```python
from build123d import *

# Parameters (mm, degrees)
SKETCH_1_W          = 100
SKETCH_1_H          = 60
EXTRUDE_1_DEPTH     = 20
SKETCH_2_W          = 90
SKETCH_2_H          = 50
CUT_EXTRUDE_1_DEPTH = 15
CUT_EXTRUDE_6_DEPTH = 200
SKETCH_9_R          = 5
CUT_EXTRUDE_7_DEPTH = 2
CUT_EXTRUDE_START   = -2
SKETCH_10_R         = 5
CUT_EXTRUDE_8_DEPTH = 2
SKETCH_11_W         = 30
SKETCH_11_H         = 3.05
EXTRUDE_2_DEPTH     = 4
SKETCH_12_W         = 30
SKETCH_12_H         = 3.05
EXTRUDE_3_DEPTH     = 4


with BuildPart() as part:
    # 草图1 → 凸台-拉伸1 (new body)
    with BuildSketch(Plane(origin=(0, 0, 0), x_dir=(1, 0, 0), z_dir=(0, 1, 0))):
        with Locations((29.550198358, -13.555421679)):
            Rectangle(SKETCH_1_W, SKETCH_1_H)
    extrude(amount=EXTRUDE_1_DEPTH)

    # 草图2 → 切除-拉伸1 (cut)
    with BuildSketch(Plane.XZ):
        with Locations((29.550198358, 13.555421679)):
            Rectangle(SKETCH_2_W, SKETCH_2_H)
    extrude(amount=-CUT_EXTRUDE_1_DEPTH, mode=Mode.SUBTRACT)

    # 草图8 → 切除-拉伸6 (cut)
    with BuildSketch(Plane.XY.offset(43.555421679)):
        with BuildLine():
            ThreePointArc((32.150198358, 10), (31.388675989, 11.838477631), (29.550198358, 12.6))
            Line((29.550198358, 12.6), (29.550198358, 7.4))
            ThreePointArc((29.550198358, 7.4), (31.388675989, 8.161522369), (32.150198358, 10))
        make_face()
        with BuildLine():
            Line((29.550198358, 7.4), (29.550198358, 12.6))
            ThreePointArc((29.550198358, 12.6), (26.950198358, 10), (29.550198358, 7.4))
        make_face()
    extrude(amount=-CUT_EXTRUDE_6_DEPTH, mode=Mode.SUBTRACT)

    # 草图9 → 切除-拉伸7 (cut)
    with BuildSketch(Plane.XY.offset(-11.444578321)):
        with Locations((29.550198358, 10)):
            Circle(SKETCH_9_R)
    extrude(amount=-CUT_EXTRUDE_7_DEPTH, mode=Mode.SUBTRACT)

    # 草图10 → 切除-拉伸8 (cut)
    with BuildSketch(Plane(origin=(0, 0, 38.555421679), x_dir=(-1, 0, 0), z_dir=(0, 0, -1)).offset(CUT_EXTRUDE_START)):
        with Locations(Location((-29.550198358, 10, 0), (0, 0, 180))):
            Circle(SKETCH_10_R)
    extrude(amount=CUT_EXTRUDE_8_DEPTH, mode=Mode.SUBTRACT)

    # 草图11 → 凸台-拉伸2 (add)
    with BuildSketch(Plane(origin=(0, 0, -16.444578321), x_dir=(-1, 0, 0), z_dir=(0, 0, -1))):
        with Locations((5.449801642, 8.475)):
            Rectangle(SKETCH_11_W, SKETCH_11_H)
        with Locations((5.449801642, 11.525)):
            Rectangle(SKETCH_11_W, SKETCH_11_H)
        with Locations((-64.550198358, 8.475)):
            Rectangle(SKETCH_11_W, SKETCH_11_H)
        with Locations((-64.550198358, 11.525)):
            Rectangle(SKETCH_11_W, SKETCH_11_H)
    extrude(amount=EXTRUDE_2_DEPTH)

    # 草图12 → 凸台-拉伸3 (add)
    with BuildSketch(Plane.XY.offset(43.555421679)):
        with Locations((-5.449801642, 11.525)):
            Rectangle(SKETCH_12_W, SKETCH_12_H)
        with Locations((-5.449801642, 8.475)):
            Rectangle(SKETCH_12_W, SKETCH_12_H)
        with Locations((64.550198358, 11.525)):
            Rectangle(SKETCH_12_W, SKETCH_12_H)
        with Locations((64.550198358, 8.475)):
            Rectangle(SKETCH_12_W, SKETCH_12_H)
    extrude(amount=EXTRUDE_3_DEPTH)


solid = part.part
```
Input: part model. Units: mm. Frame: model coordinates. A direction names the side the tool comes from. Coordinates: 2 decimals unless noted, no trailing zeros. Write each loop counter-clockwise with the first axis right and the second up, starting at its lowest first coordinate (ties: lowest second). Pieces come first, ordered by that corner, then holes. Notation, with made-up numbers: (65.25, 79.5) - (74.25, 79.5) arc R3 cw to (74.25, 84.5) - close; hole circle Ø3 at (24, 41.5). An arc over 180 degrees is marked (long way). Put each result on its own line as item: value. Start each with the question number.
1) Cut plane C-C (x = 61). Return the cut outline in (y, z), plus the area to 3 significant figures.
2) Reachability of faces 1 (the face through (64, 6.95, 46)), 2 (the face through (9.55, 10, -18)), 3 (the face through (29, 4, -11.445)) from +Z, -Z, +X, -X, +Y, -Y: full face, straight path, thin tool, end or side. Return the list, or none.
3) Mould query, pull axis Y, two halves, no side actions, for faces 4 (the face through (64, 13.05, 46)), 5 (the face through (32, 8, -13.445)), 6 (the face through (-20.45, 10, 14)), 7 (the face through (26, 0, 40)). Classes: pulls with the +Y half, pulls with the -Y half, needs draft (parallel to the pull), parting line crosses it, or undercut.
4) Ray query, L1, parallel to X at y = 10, z = -12.05; L2, parallel to Z at x = -9.5, y = 3; L3, parallel to X at y = 6.5, z = 15. Return the intervals inside material, ascending.
5) Contact query for flat-ended pins moving along their axis: pin 1 (4.5 mm diameter, centred on x = 15.5, y = 8.5, fed in from +Z); pin 2 (2 mm diameter, centred on x = -0.5, y = 5.5, fed in from -Z); pin 3 (12 mm diameter, centred on x = 66, y = 14.5, fed in from +Z); pin 4 (1.2 mm diameter, centred on x = -7.5, z = -18, fed in from +Y). Output: stop coordinate, or through.
6) Cut plane B-B (z = -0.5). Return the cut outline in (x, y), plus the area to 3 significant figures.
7) Cut plane D-D (y = 16.25). Return the cut outline in (x, z).
Resolved:
1. outline: (0, -16.44) - (6.95, -16.44) - (6.95, -20.44) - (13.05, -20.44) - (13.05, -16.44) - (20, -16.44) - (20, 43.56) - (13.05, 43.56) - (13.05, 47.56) - (6.95, 47.56) - (6.95, 43.56) - (0, 43.56) - (0, 38.56) - (15, 38.56) - (15, -11.44) - (0, -11.44) - close
1. area: 499 mm2
2. face 1: +Z, +X, -X, -Y
2. face 2: -Z, +Y, -Y
2. face 3: -Y
3. face 4: pulls with the +Y half
3. face 5: undercut
3. face 6: needs draft
3. face 7: pulls with the -Y half
4. L1: x = -20.45 to 24.55, 34.55 to 79.55
4. L2: z = -16.44 to -11.44, 38.56 to 43.56
4. L3: x = -20.45 to -15.45, 74.55 to 79.55
5. pin 1: stops at z = 43.56
5. pin 2: stops at z = -16.44
5. pin 3: stops at z = 47.56
5. pin 4: stops at y = 13.05
6. outline: (-20.45, 0) - (-15.45, 0) - (-15.45, 15) - (74.55, 15) - (74.55, 0) - (79.55, 0) - (79.55, 20) - (-20.45, 20) - close
6. area: 650 mm2
7. outline: (-20.45, -16.44) - (79.55, -16.44) - (79.55, 43.56) - (-20.45, 43.56) - close
